from build123d import *

# Parameters (mm, degrees)
CHAMFER1_SIZE      = 1
CHAMFER1_SIZE2     = 2
SHELL1_T           = 1.25
SKETCH3_R          = 3.318
CUT_EXTRUDE1_DEPTH = 2.54


with BuildPart() as part:
    # Sketch1 → Revolve1 (revolve)
    with BuildSketch(Plane(origin=(0, 0, 0), x_dir=(0, 0, -1), z_dir=(1, 0, 0))):
        with BuildLine():
            Line((0, 0), (95, 0))
            Line((95, 0), (95, 5.08))
            Line((95, 5.08), (84.042781462, 5.08))
            ThreePointArc((84.042781462, 5.08), (82.450318528, 5.336053296), (81.018389209, 6.078400864))
            ThreePointArc((81.018389209, 6.078400864), (71.521540522, 11.001802069), (60.96, 12.7))
            Line((60.96, 12.7), (12.7, 12.7))
            ThreePointArc((12.7, 12.7), (3.719743879, 8.980256121), (0, 0))
        make_face()
    revolve(axis=Axis((0, 0, 0), (0, 0, -1)))

    # Chamfer1
    chamfer1_edges = [part.edges().sort_by_distance(p)[0] for p in [
        (0, -5.08, -95),
    ]]
    chamfer1_side = [part.faces().sort_by_distance(p)[0] for p in [
        (0, 0, -95),
    ]]
    chamfer(chamfer1_edges, length=CHAMFER1_SIZE, length2=CHAMFER1_SIZE2, reference=chamfer1_side[0])

    # Shell1 (no face opened: a closed hollow body)
    add(offset(amount=-SHELL1_T, mode=Mode.PRIVATE), mode=Mode.SUBTRACT)

    # Sketch3 → Cut-Extrude1 (cut)
    with BuildSketch(Plane(origin=(0, 0, -95), x_dir=(-1, 0, 0), z_dir=(0, 0, -1))):
        Circle(SKETCH3_R)
    extrude(amount=-CUT_EXTRUDE1_DEPTH, mode=Mode.SUBTRACT)


solid = part.part
Work out the finished part from the listing and answer in its coordinate system (mm). A direction names the side the tool comes from. Round coordinates to 2 decimals unless told otherwise and drop trailing zeros. Loops run counter-clockwise (first coordinate to the right, second up) from the corner with the lowest first, then second, coordinate; pieces in that order, holes last. Notation, with made-up numbers: (11.5, -35.75) - (31.5, -35.75) arc R3 ccw to (31.5, -30.75) - close; hole circle Ø4 at (-1.75, 89). An arc over 180 degrees is marked (long way). Use one line per item in the form item = value. Start each with the question number.
(1) Determine the mould class of faces 1 (the face through (-3, -2, -95)), 2 (the face through (3.797, -0.499, -88.313)), 3 (the face through (-12.4, -2.75, -36.49)) for opening direction X: +X half, -X half, draft (parallel to the pull), parting line (faces both ways), or undercut.
(2) Which of the six approach directions +Z, -Z, +X, -X, +Y, -Y give full straight-line access (tool end or side, diameter ignored) to faces 4 (the face through (-11.18, -2.48, -36.49)), 5 (the face through (5.037, -0.661, -88.459))?
(3) Consider line 1 (X direction, y = 0, z = -87.5); line 2 (X direction, y = 0, z = -94.7); line 3 (Y direction, x = -7.5, z = -40.5). Determine where each line is inside the solid, lowest interval first.
(4) Flat-ended cylindrical pins translate along their axes: P1, Ø3, axis at x = 9, z = -35, coming from the -Y side; P2, Ø4, axis at y = -2, z = -21.5, coming from the -X side; P3, Ø12, axis at x = -9, z = -19, coming from the -Y side; P4, Ø1, axis at x = -6, y = 2, coming from the +Z side. Find the tip coordinate at first contact, or state that the pin passes through.
(5) Find section A-A on z = -52. Determine the outline of the cut face in (x, y), and give its area (3 significant figures).
Answer list:
q1.face_1 = draft
q1.face_2 = undercut
q1.face_3 = parting line
q2.face_4 = none
q2.face_5 = -Z
q3.line_1 = -5.08 to -3.83, 3.83 to 5.08
q3.line_2 = -4.23 to -3.32, 3.32 to 4.23
q3.line_3 = -10.25 to -8.65, 8.65 to 10.25
q4.P1 = -10.25
q4.P2 = -12.7
q4.P3 = -12.34
q4.P4 = -1.41
q5.outline = circle Ø25.4 at (0, 0); hole circle Ø22.9 at (0, 0)
q5.area = 94.8 mm^2
